Work out the finished part from the listing and answer in its coordinate system (mm). A direction names the side the tool comes from. Give positions to 0.01 mm unless a question says otherwise; leave off trailing zeros. Order: outer loops, then holes, each group sorted by start corner. A loop starts at its lowest first (then second) coordinate and runs counter-clockwise, first axis right, second up. Notation, with made-up numbers: (42, -28) - (79, -28) arc R17 cw to (79, -11) - close; hole circle Ø1 at (52.5, 7.25). An arc over 180 degrees is marked (long way). Return JSON: item names as keys, results as strings. Group by question number.
from build123d import *

# Parameters (mm, degrees)
BOSS_EXTRUDE1_DEPTH = 4


with BuildPart() as part:
    # Sketch1 → Boss-Extrude1 (new body)
    with BuildSketch(Plane.XY):
        Polygon((-20.165601387, 14.911355428), (-17.538478408, 17.927681812), (20.165601387, -14.911355428), (17.538478408, -17.927681812), align=None)
        Polygon((-17.538478408, -17.927681812), (-20.165601387, -14.911355428), (17.538478408, 17.927681812), (20.165601387, 14.911355428), align=None)
    extrude(amount=BOSS_EXTRUDE1_DEPTH)


solid = part.part
1. A tool of negligible diameter and unlimited length cuts with its end or side. For faces 4 (the flat face through (-11.486, 7.351, 1.972)), 5 (the flat face through (-8.892, 10.397, 1.972)), 6 (the flat face through (11.725, 7.56, 1.972)), from which of +Z, -Z, +X, -X, +Y, -Y can it reach the whole face along a straight path? Write none if from no direction.
2. The part is cut by section B-B (x = 4). Give the vertices of the cut face in (y, z), and give its area (3 significant figures).
3. Each of these flat-tipped pins is pushed along its axis until it touches: pin 1 (5 mm diameter, centred on x = -9.5, y = 2, fed in from +Z); pin 2 (2 mm diameter, centred on x = 8.5, z = 1, fed in from +Y); pin 3 (1 mm diameter, centred on y = -2.5, z = 3.5, fed in from -X); pin 4 (1 mm diameter, centred on y = 8, z = 3.5, fed in from -X). Where does it stop, or does it pass through?
4. Determine the mould class of faces 1 (the flat face through (-18.834, -16.441, 1.972)), 2 (the flat face through (11.486, -7.351, 1.972)), 3 (the flat face through (-18.87, 16.4, 1.97)) for opening direction Y: released by +Y, released by -Y, zero draft, split by the parting line, or undercut.
5. The part is cut by section D-D (x = -2). Give the vertices of the cut face in (y, z).
6. Consider probe 1 along Y at (x, z) = (18, 2.6); probe 2 along Y at (x, z) = (6, 2.1); probe 3 along X at (y, z) = (11, 1.05). Determine where each line is inside the solid, lowest interval first. Write a range as from..to.
7. The part is cut by section C-C (z = 3.15). Give the vertices of the cut face in (x, y).
8. The part is cut by section A-A (y = 10). Give the vertices of the cut face in (x, z).
Answers:
{
 "1": {"face 4": "+Z, -Z, -X", "face 5": "+Z, -Z, +Y", "face 6": "+Z, -Z, +X"},
 "2": {"outline": "(-6.14, 0) - (-0.83, 0) - (-0.83, 4) - (-6.14, 4) - close; (0.83, 0) - (6.14, 0) - (6.14, 4) - (0.83, 4) - close", "area": "42.4 mm^2"},
 "3": {"pin 1": "passes through", "pin 2": "stops at y = 10.93", "pin 3": "stops at x = -6.49", "pin 4": "stops at x = -12.8"},
 "4": {"face 1": "released by -Y", "face 2": "undercut", "face 3": "released by +Y"},
 "5": {"outline": "(-4.39, 0) - (4.39, 0) - (4.39, 4) - (-4.39, 4) - close"},
 "6": {"probe 1": "y = -17.4..-13.03, 13.03..17.4", "probe 2": "y = -7.88..-2.57, 2.57..7.88", "probe 3": "x = -15.67..-9.58, 9.58..15.67"},
 "7": {"outline": "(-20.17, -14.91) - (-17.54, -17.93) - (0, -2.65) - (17.54, -17.93) - (20.17, -14.91) - (3.05, 0) - (20.17, 14.91) - (17.54, 17.93) - (0, 2.65) - (-17.54, 17.93) - (-20.17, 14.91) - (-3.05, 0) - close"},
 "8": {"outline": "(-14.53, 0) - (-8.44, 0) - (-8.44, 4) - (-14.53, 4) - close; (8.44, 0) - (14.53, 0) - (14.53, 4) - (8.44, 4) - close"}
}
